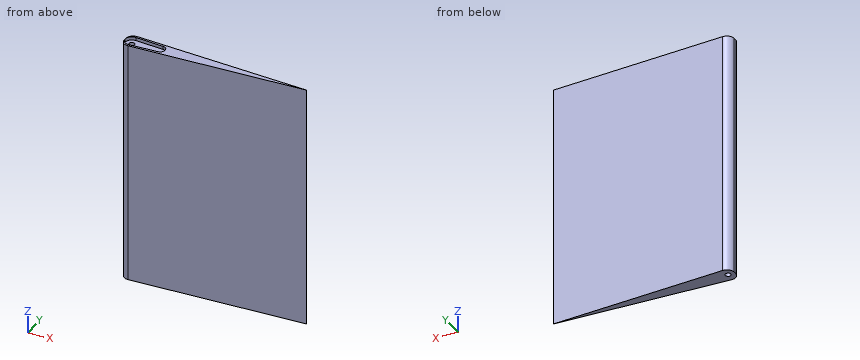
Autodesk Inventor part; units mm, degrees
ref_plane "YZ Plane" through (0, 0, 0) normal (1, 0, 0) x (0, 1, 0)
ref_plane "XZ Plane" through (0, 0, 0) normal (0, 1, 0) x (-1, 0, 0)
ref_plane "XY Plane" through (0, 0, 0) normal (0, 0, 1) x (1, 0, 0)
sketch "Sketch1" plane through (0, 0, 0) normal (0, 0, 1) x (1, 0, 0)
  line L0 (357.0794, 41.0884) -> (357.0794, 43.1077)
  line L1 (362.4131, 48.1813) -> (484.0794, 42.098)
  line L2 (484.0794, 42.098) -> (362.4131, 36.0147)
  arc A0 (362.4131, 48.1813) -> (357.0794, 43.1077) centre (362.1594, 43.1077) ccw
  arc A1 (357.0794, 41.0884) -> (362.4131, 36.0147) centre (362.1594, 41.0884) ccw
  point P0 (357.0794, 35.748)
  point P1 (357.0794, 48.448)
  dimension "d0" = 127
  dimension "d1" = 12.7
  dimension "d2" = 5.08
extrude "Extrusion1" add sketch "Sketch1" along normal blind 170.0022
sketch "Sketch2" plane through (0, 0, 170.0022) normal (0, 0, 1) x (1, 0, 0)
  arc A0 (362.1294, 46.8881) -> (362.4259, 37.4357) centre (361.8271, 42.1478) ccw
  arc A1 (381.5771, 38.6478) -> (381.5771, 45.6478) centre (381.5771, 42.1478) ccw
  arc A2 (381.5771, 38.6478) -> (381.5771, 45.6478) centre (381.5771, 42.1478) ccw
  line L0 (361.8271, 37.3978) -> (381.5771, 38.6478)
  line L1 (381.5771, 45.6478) -> (362.1294, 46.8881)
  point P0 (0, 0)
  point P1 (367.7181, 34.9628)
  point P2 (367.4202, 34.9628)
  point P3 (357.0794, 41.9988)
  point P4 (356.8779, 76.4339)
  point P5 (354.6232, 35.4991)
  point P6 (354.3254, 35.4991)
extrude "Extrusion2" cut sketch "Sketch2" against normal blind 2.25 contours L1 A1 L0 A0
sketch "Sketch3" plane through (0, 0, 167.7522) normal (0, 0, 1) x (1, 0, 0)
  line L0 (357.0794, 41.9988) -> (357.0794, 42.2967)
  arc A0 (357.0794, 41.9988) -> (361.8271, 37.3978) centre (361.8271, 42.1478) ccw
  line L1 (381.5771, 38.6478) -> (361.8271, 37.3978)
  arc A1 (381.5771, 38.6478) -> (381.5771, 45.6478) centre (381.5771, 42.1478) ccw
  line L2 (362.1294, 46.8881) -> (381.5771, 45.6478)
  arc A2 (362.1294, 46.8881) -> (357.0794, 42.2967) centre (361.8271, 42.1478) ccw
  circle A3 centre (361.8271, 42.1478) radius 1.905
  point P0 (0, 0)
  dimension "d7" = 3.81
extrude "Extrusion3" cut sketch "Sketch3" against normal blind 170.18 contours A3
properties part number "ElevatorV2"
Source: CAD feature listing. Evaluate the final solid. Frame: model axes, mm. Round coordinates to 2 decimals unless told otherwise and drop trailing zeros. Loops run counter-clockwise (first coordinate to the right, second up) from the corner with the lowest first, then second, coordinate; pieces in that order, holes last.
(1) Section query C-C (x = 428.5). Output: boundary loops of the cut face in (y, z), and give its area (3 significant figures).
From the geometry:
outline: (39.32, 0) - (44.88, 0) - (44.88, 170) - (39.32, 170) - close
area: 945 mm2
(2) Material intervals for probe 1 along Y at (x, z) = (478.5, 95.5); probe 2 along Y at (x, z) = (449.5, 18.5), sorted ascending.
From the geometry:
probe 1: y = 41.82 to 42.38
probe 2: y = 40.37 to 43.83
(3) Contact query for flat-ended pins moving along their axis: pin 1 Ø1 at (y, z) = (39, 129.5) entering from -X; pin 2 Ø8 at (x, z) = (412.5, 49) entering from -Y; pin 3 Ø1.5 at (x, z) = (413, 114.5) entering from +Y. Output: stop coordinate, or through.
From the geometry:
pin 1: stops at x = 357.33
pin 2: stops at y = 38.32
pin 3: stops at y = 45.69
(4) Section query D-D (x = 442). Output: boundary loops of the cut face in (y, z).
From the geometry:
outline: (39.99, 0) - (44.2, 0) - (44.2, 170) - (39.99, 170) - close
(5) Section query B-B (z = 67). Output: boundary loops of the cut face in (x, y) (3 decimals).
From the geometry:
outline: (357.079, 41.088) arc R5.08 ccw to (362.413, 36.015) - (484.079, 42.098) - (362.413, 48.181) arc R5.08 ccw to (357.079, 43.108) - close; hole circle Ø3.81 at (361.827, 42.148)
(6) Section query A-A (x = 366.5). Output: boundary loops of the cut face in (y, z), and give its area (3 significant figures).
From the geometry:
outline: (36.22, 0) - (47.98, 0) - (47.98, 170) - (46.61, 170) - (46.61, 167.75) - (37.69, 167.75) - (37.69, 170) - (36.22, 170) - close
area: 1,980 mm2
